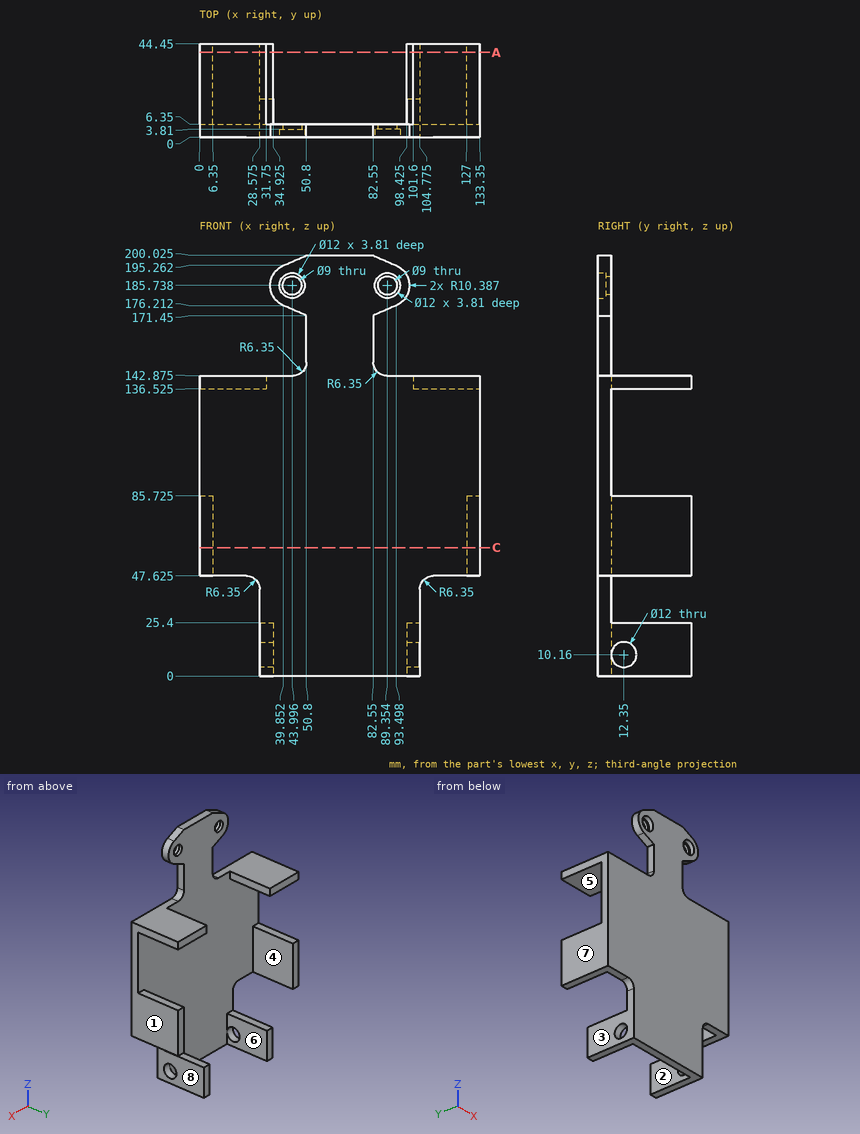
Here's the drawing with two shaded views (mm, measured from the low corner). I have some questions. A direction names the side the tool comes from. Give positions to 0.01 mm unless a question says otherwise; leave off trailing zeros. Order: outer loops, then holes, each group sorted by start corner. A loop starts at its lowest first (then second) coordinate and runs counter-clockwise, first axis right, second up. Notation, with made-up numbers: (61, 56) -> (83, 56) arc R21 ccw to (83, 93) -> close; hole circle Ø4 at (62.25, 35.25). An arc over 180 degrees is marked (long way). One line per item, written item: value. Start each with the question number.
1. Imagine slicing it at A-A, the plane y = 40.5. Count the separate pieces of the cut face and the enclosed holes in it, plus the area to 3 significant figures.
2. Will these pins go through, and if not, where does the flat tip stop? pin 1 Ø12.5 at (y, z) = (26.5, 17) entering from +X (1 decimal); pin 2 Ø1.9 at (y, z) = (2, 164.5) entering from -X; pin 3 Ø12.5 at (y, z) = (25, 31) entering from -X (1 decimal).
3. We'd pull the mould along X, two halves only. Please class the marked faces 6, 7 and 8: released by +X, released by -X, zero draft, split by the parting line, or undercut.
4. For the marked faces 1, 2, 3, 4 and 5, which set-ups out of +Z, -Z, +X, -X, +Y, -Y let a thin tool reach every point of the face, with its end or its side?
5. I need wall thicknesses on probe 1 along Y at (x, z) = (32.75, 10.16); probe 2 along X at (y, z) = (26.5, 14.5) (1 decimal); probe 3 along X at (y, z) = (20, 55). Which ranges of each line are inside material? Lowest first, please. Write a range as from..to.
6. Imagine slicing it at C-C, the plane z = 61. List the corners of the cut face in (x, y) for me, plus the area to 3 significant figures.
Values follow:
1. separate pieces: 6
1. enclosed holes: 0
1. area: 1,210 mm2
2. pin 1: stops at x = 104.8
2. pin 2: stops at x = 50.8
2. pin 3: stops at x = 28.6
3. face 6: undercut
3. face 7: released by -X
3. face 8: released by +X
4. face 1: +Z, -Z, +X, +Y, -Y
4. face 2: +Z, -Z, +Y
4. face 3: -Z, -X, +Y, -Y
4. face 4: -Z, +Y
4. face 5: +X, -X, +Y
5. probe 1: y = 0..6.35, 18.35..44.45
5. probe 2: x = 28.6..34.9, 98.4..104.8
5. probe 3: x = 0..6.35, 127..133.35
6. outline: (0, 0) -> (133.35, 0) -> (133.35, 44.45) -> (127, 44.45) -> (127, 6.35) -> (6.35, 6.35) -> (6.35, 44.45) -> (0, 44.45) -> close
6. area: 1,330 mm2
